Check sheet for the modelled part. Datum: model origin and axes. Units: mm. Round coordinates to 2 decimals unless told otherwise and drop trailing zeros. Order: outer loops, then holes, each group sorted by start corner. A loop starts at its lowest first (then second) coordinate and runs counter-clockwise, first axis right, second up.
(1) Depth check by flat-ended pin: pin 1 (6.5 mm diameter, centred on y = -5, z = 9.5, fed in from -X); pin 2 (3 mm diameter, centred on x = -11.5, z = -41, fed in from +Y). Enter the tip coordinate at first touch or a pass-through.
(2) Thickness scan on probe 1 along Z at (x, y) = (21, -5.5); probe 2 along Y at (x, z) = (38, -41); probe 3 along X at (y, z) = (-2.75, 47.5). Record the ranges inside material, lowest first.
(3) Sectioned sample at D-D, the plane z = 37.5. Enter the section's corners in (x, y), and give its area (3 significant figures).
(4) Sectioned sample at A-A, the plane y = -2. Enter the section's corners in (x, z).
(5) Sectioned sample at B-B, the plane x = -6.5. Enter the section's corners in (y, z), and give its area (3 significant figures).
(6) Sectioned sample at C-C, the plane z = 25.4. Enter the section's corners in (x, y), and give its area (3 significant figures).
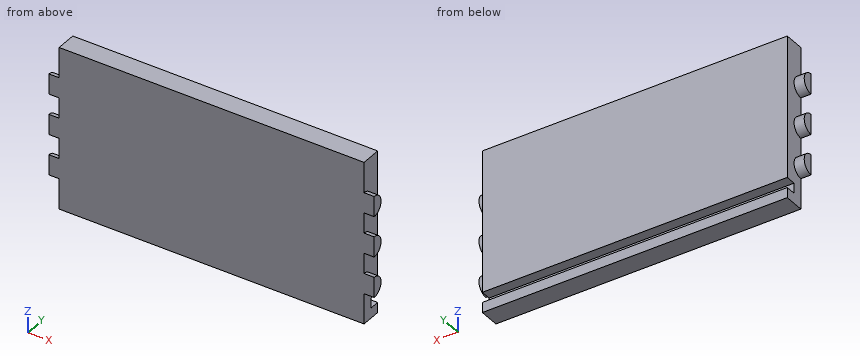
```python
from build123d import *

# Parameters (mm, degrees)
F0_W     = 190.5
F0_H     = 88.9
F0_H_2   = 6.35
F1_DEPTH = 12.7
F2_DEPTH = 6.35
F4_DEPTH = 6.35
F6_DEPTH = 6.35


with BuildPart() as f1:
    # F0 (on Front) → F1 (new body)
    with BuildSketch(Plane.XZ):
        Polygon((103.884577, -50.8), (103.884577, 50.8), (97.534577, 50.8), (97.534577, -38.1), (97.534577, -44.45), (97.534577, -50.8), align=None)
        with Locations((2.284577, 6.35)):
            Rectangle(F0_W, F0_H)
        Polygon((-92.965423, -38.1), (-92.965423, 50.8), (-99.315423, 50.8), (-99.315423, -50.8), (-92.965423, -50.8), (-92.965423, -44.45), align=None)
        with Locations((2.284577, -47.625)):
            Rectangle(F0_W, F0_H_2)
        with Locations((2.284577, -41.275)):
            Rectangle(F0_W, F0_H_2)
    extrude(amount=F1_DEPTH)

    # F0 (on Front) → F2 (cut)
    with BuildSketch(Plane.XZ):
        with Locations((2.284577, -41.275)):
            Rectangle(F0_W, F0_H_2)
    extrude(amount=F2_DEPTH, mode=Mode.SUBTRACT)

    # F3 (on face) → F4 (cut)
    with BuildSketch(Plane(origin=(-99.315423, 0, 0), x_dir=(0, -1, 0), z_dir=(-1, 0, 0))):
        with BuildLine():
            ThreePointArc((12.7, 19.05), (6.35, 25.4), (12.7, 31.75))
            Line((12.7, 31.75), (12.7, 50.8))
            Line((12.7, 50.8), (0, 50.8))
            Line((0, 50.8), (0, -50.8))
            Line((0, -50.8), (12.7, -50.8))
            Line((12.7, -50.8), (12.7, -31.75))
            ThreePointArc((12.7, -31.75), (6.35, -25.4), (12.7, -19.05))
            Line((12.7, -19.05), (12.7, -6.35))
            ThreePointArc((12.7, -6.35), (6.35, 0), (12.7, 6.35))
            Line((12.7, 6.35), (12.7, 19.05))
        make_face()
    extrude(amount=-F4_DEPTH, mode=Mode.SUBTRACT)

    # F5 (on face) → F6 (cut)
    with BuildSketch(Plane.YZ.offset(103.884577)):
        with BuildLine():
            ThreePointArc((-12.7, 31.75), (-6.35, 25.4), (-12.7, 19.05))
            Line((-12.7, 19.05), (-12.7, 6.35))
            ThreePointArc((-12.7, 6.35), (-6.35, 0), (-12.7, -6.35))
            Line((-12.7, -6.35), (-12.7, -19.05))
            ThreePointArc((-12.7, -19.05), (-6.35, -25.4), (-12.7, -31.75))
            Line((-12.7, -31.75), (-12.7, -50.8))
            Line((-12.7, -50.8), (0, -50.8))
            Line((0, -50.8), (0, 50.8))
            Line((0, 50.8), (-12.7, 50.8))
            Line((-12.7, 50.8), (-12.7, 31.75))
        make_face()
    extrude(amount=-F6_DEPTH, mode=Mode.SUBTRACT)


solid = f1.part
```
Derived:
1. pin 1: stops at x = -92.97
1. pin 2: stops at y = -6.35
2. probe 1: z = -50.8 to -44.45, -38.1 to 50.8
2. probe 2: y = -12.7 to -6.35
2. probe 3: x = -92.97 to 97.53
3. outline: (-92.97, -12.7) - (97.53, -12.7) - (97.53, 0) - (-92.97, 0) - close
3. area: 2,420 mm2
4. outline: (-92.97, -50.8) - (97.53, -50.8) - (97.53, -44.45) - (-92.97, -44.45) - close; (-92.97, -38.1) - (97.53, -38.1) - (97.53, 50.8) - (-92.97, 50.8) - close
5. outline: (-12.7, -50.8) - (0, -50.8) - (0, -44.45) - (-6.35, -44.45) - (-6.35, -38.1) - (0, -38.1) - (0, 50.8) - (-12.7, 50.8) - close
5. area: 1,250 mm2
6. outline: (-99.32, -12.7) - (103.88, -12.7) - (103.88, -6.35) - (97.53, -6.35) - (97.53, 0) - (-92.97, 0) - (-92.97, -6.35) - (-99.32, -6.35) - close
6. area: 2,500 mm2
